Part print with two shaded views. Sizes in mm from the minimum x, y, z corner. A direction names the side the tool comes from. Give positions to 0.01 mm unless a question says otherwise; leave off trailing zeros. Order: outer loops, then holes, each group sorted by start corner. A loop starts at its lowest first (then second) coordinate and runs counter-clockwise, first axis right, second up. Notation, with made-up numbers: M -29.5,-19 L -24.5,-19 A16 ccw -24.5,10 Z; hole C 25.25,35 d10. An arc over 180 degrees is marked long. Answer as CSV lines item,"result".
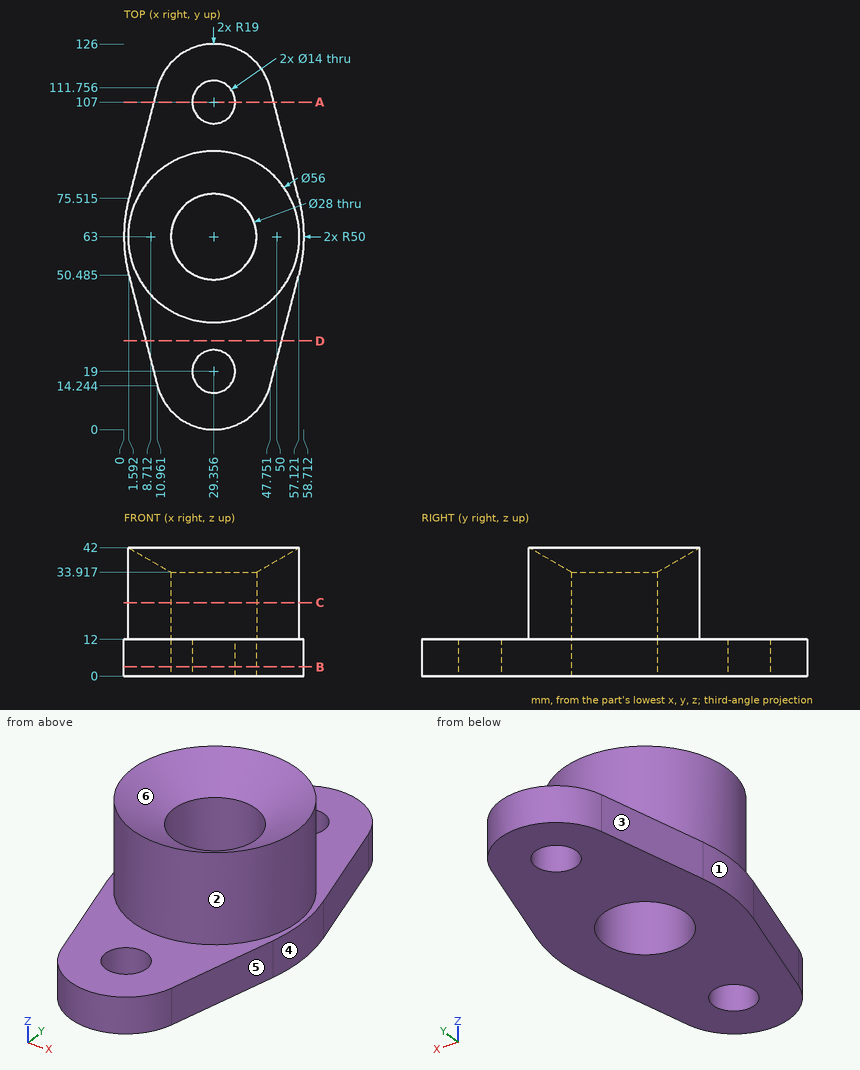
Item 1: Band-saw the part on D-D (y = 29). Give the cut face in (x, z).
Geometry says:
outline,"M 7.15,0 L 51.57,0 L 51.57,12 L 7.15,12 Z"
Item 2: 3-axis set-ups, long thin cutter, end or side, ignore diameter. For the marked faces 1 and 2: which of +Z, -Z, +X, -X, +Y, -Y reach the whole face in a straight line?
Geometry says:
face 1,"+Z, -Z, -X"
face 2,"+Z"
Item 3: Probe line 1 along X through (y, z) = (63, 16); line 2 along Z through (x, y) = (46, 88.5); line 3 along Y through (x, z) = (37, 18.5) (1 decimal). List the from-to ranges inside material, lowest first. Write a range as from..to.
Geometry says:
line 1,"x = 1.36..15.36, 43.36..57.36"
line 2,"z = 0..12"
line 3,"y = 36.1..51.3, 74.7..89.9"
Item 4: Drop flat-ended pins along their axis: pin 1 (8 mm diameter, centred on x = 6.5, z = 17, fed in from +Y); pin 2 (1 mm diameter, centred on x = 19.5, z = 35.5, fed in from +Y); pin 3 (2 mm diameter, centred on x = 42, z = 19.5, fed in from -Y) (1 decimal). Give the stop position or say it passes through.
Geometry says:
pin 1,"stops at y = 83.7"
pin 2,"stops at y = 89.39"
pin 3,"stops at y = 37.5"
Item 5: Band-saw the part on C-C (z = 24). Give the cut face in (x, y).
Geometry says:
outline,"C 29.36,63 d56; hole C 29.36,63 d28"
Item 6: Pull direction Y, two halves, no side cores. Call the marked faces 3, 4, 5 and 6: released by +Y, released by -Y, zero draft, split by the parting line, or undercut.
Geometry says:
face 3,"released by +Y"
face 4,"split by the parting line"
face 5,"released by -Y"
face 6,"undercut"
Item 7: Band-saw the part on B-B (z = 3). Give the cut face in (x, y) (1 decimal).
Geometry says:
outline,"M 1.6,50.5 L 11,14.2 A19 ccw 47.8,14.2 L 57.1,50.5 A50 ccw 57.1,75.5 L 47.8,111.8 A19 ccw 11,111.8 L 1.6,75.5 A50 ccw Z; hole C 29.4,63 d28; hole C 29.4,19 d14; hole C 29.4,107 d14"
Item 8: Band-saw the part on A-A (y = 107). Give the cut face in (x, z), and give its area (3 significant figures).
Geometry says:
outline,"M 9.73,0 L 22.36,0 L 22.36,12 L 9.73,12 Z; M 36.36,0 L 48.98,0 L 48.98,12 L 36.36,12 Z"
area,"303 mm2"
